The listing builds one solid part. Answer for the finished solid, in the listing's coordinates (mm). A direction names the side the tool comes from. Coordinates: 2 decimals unless noted, no trailing zeros. Loops run counter-clockwise (first coordinate to the right, second up) from the corner with the lowest first, then second, coordinate; pieces in that order, holes last. Notation, with made-up numbers: (32, 44) - (83, 44) arc R20 ccw to (83, 64) - close; hole circle Ø4 at (-8.5, 17.5). An arc over 180 degrees is marked (long way). One line per question, with ' | ' between items.
Autodesk Inventor part; units mm, degrees
ref_plane "YZ Plane" through (0, 0, 0) normal (1, 0, 0) x (0, 1, 0)
ref_plane "XZ Plane" through (0, 0, 0) normal (0, 1, 0) x (-1, 0, 0)
ref_plane "XY Plane" through (0, 0, 0) normal (0, 0, 1) x (1, 0, 0)
sketch "Skizze1" plane through (0, 0, 0) normal (0, 0, 1) x (1, 0, 0)
  line L0 (49.5001, 248.3761) -> (-49.5001, 248.3761)
  line L1 (49.5001, 95.1751) -> (49.5001, 248.3761)
  line L2 (-49.5001, 248.3761) -> (-49.5001, 95.1751) construction
  line L3 (-49.5001, 95.1751) -> (49.5001, 95.1751) construction
  line L4 (49.5001, 95.1751) -> (-20.5915, 95.1751)
  line L5 (-20.5915, 95.1751) -> (-49.5001, 124.0836)
  line L6 (-49.5001, 124.0836) -> (-49.5001, 248.3761)
  line L7 (-39.5001, 238.3761) -> (39.5001, 238.3761)
  line L8 (39.5001, 238.3761) -> (39.5001, 105.1751)
  line L9 (39.5001, 105.1751) -> (-19.2778, 105.1751)
  line L10 (-19.2778, 105.1751) -> (-39.5001, 125.3973)
  line L11 (-39.5001, 125.3973) -> (-39.5001, 238.3761)
  circle A0 centre (44.5001, 243.3761) radius 2.5
  circle A1 centre (-44.5001, 243.3761) radius 2.5
  circle A2 centre (-44.5001, 171.4345) radius 2.5
  circle A3 centre (44.5001, 171.4345) radius 2.5
  circle A4 centre (44.5001, 100.1751) radius 2.5
  circle A5 centre (-20.9666, 110.5265) radius 1.75
  circle A6 centre (-24.6237, 114.0565) radius 1.75
  circle A7 centre (-44.8001, 100.0237) radius 1.75
  circle A8 centre (-29.7001, 100.0237) radius 1.75
  point P0 (0, 0)
  dimension "d0" = 135
  dimension "d1" = 8
  dimension "d3" = 10
  dimension "d4" = 10
  dimension "d5" = 10
  dimension "d6" = 10
  dimension "d22" = 2.5
extrude "Extrusion1" add sketch "Skizze1" along normal blind 1.5 contours L1 L4 L5 L6 L0 | A0 | A1 | A2 | A3 | A4
sketch "Skizze2" plane through (0, 0, 0) normal (0, 0, -1) x (-1, 0, 0)
  circle A0 centre (-44.5001, 100.1751) radius 2.5
  circle A1 centre (-44.5001, 171.4345) radius 2.5
  circle A2 centre (-44.5001, 243.3761) radius 2.5
  circle A3 centre (40.1569, 120.3973) radius 2.5
  circle A4 centre (44.5001, 171.4345) radius 2.5
  circle A5 centre (44.5001, 243.3761) radius 2.5
  circle A6 centre (-44.5001, 100.1751) radius 2.4
  circle A7 centre (-44.5001, 171.4345) radius 2.4
  circle A8 centre (-44.5001, 243.3761) radius 2.4
  circle A9 centre (44.5001, 243.3761) radius 2.4
  circle A10 centre (44.5001, 171.4345) radius 2.4
  circle A11 centre (40.1569, 120.3973) radius 2.4
  dimension "d23" = 0.1
  dimension "d24" = 4.8
  dimension "d25" = 4.8
  dimension "d26" = 4.8
  dimension "d27" = 4.8
  dimension "d28" = 4.8
  dimension "d29" = 4.8
extrude "Extrusion2" add sketch "Skizze2" along normal blind 2.6 contours A6 | A7 | A8 | A9 | A10 | A11
sketch "Skizze3" plane through (0, 0, 0) normal (0, 0, -1) x (-1, 0, 0)
  line L0 (-49.5001, 95.1751) -> (-49.5001, 248.3761)
  line L1 (-39.5001, 238.3761) -> (-39.5001, 105.1751)
  line L2 (-49.5001, 135.1751) -> (-39.5001, 135.1751)
  line L3 (-39.5001, 135.1751) -> (-39.5001, 145.1751)
  line L4 (-39.5001, 145.1751) -> (-49.5001, 145.1751)
  line L5 (-49.5001, 145.1751) -> (-49.5001, 135.1751)
  line L6 (39.5001, 238.3761) -> (39.5001, 125.3973)
  line L7 (49.5001, 248.3761) -> (49.5001, 124.0836)
  line L8 (39.5001, 135.1751) -> (49.5001, 135.1751)
  line L9 (49.5001, 135.1751) -> (49.5001, 145.1751)
  line L10 (49.5001, 145.1751) -> (39.5001, 145.1751)
  line L11 (39.5001, 145.1751) -> (39.5001, 135.1751)
  line L12 (39.5001, 125.3973) -> (19.2778, 105.1751)
  line L13 (20.692, 106.5893) -> (26.3489, 100.9324)
  line L14 (49.5001, 124.0836) -> (20.5915, 95.1751)
  line L15 (26.3489, 100.9324) -> (33.42, 108.0035)
  line L16 (33.42, 108.0035) -> (27.7631, 113.6604)
  line L17 (27.7631, 113.6604) -> (20.692, 106.5893)
  line L18 (20.5915, 95.1751) -> (-49.5001, 95.1751)
  point P0 (0, 0)
  dimension "d11" = 10
  dimension "d12" = 10
  dimension "d13" = 10
  dimension "d14" = 0
  dimension "d15" = 40
  dimension "d16" = 2
extrude "Extrusion3" cut sketch "Skizze3" against normal blind 1 contours L0 L4 L1 L2 | L13 L12 L16 L14 | L8 L6 L10 L7
equation "\"d4\" = d3"
equation "\"d5\" = d3"
equation "\"d6\" = d3"
equation "\"d25\" = d24"
equation "\"d26\" = d24"
equation "\"d27\" = d24"
equation "\"d28\" = d24"
equation "\"d29\" = d24"
equation "\"d12\" = d11"
equation "\"d13\" = d11"
properties part number "Backplate_V2"
Item 1: Each of these flat-tipped pins is pushed along its axis until it touches: pin 1 Ø6.5 at (x, y) = (-34.5, 118.5) entering from -Z; pin 2 Ø3 at (x, y) = (-46.5, 138.5) entering from -Z; pin 3 Ø0.5 at (x, z) = (-46, 0.5) entering from -Y. Where does it stop, or does it pass through?
Taken from the geometry:
pin 1: stops at z = 0 | pin 2: stops at z = 1 | pin 3: stops at y = 120.33
Item 2: Find section C-C, the plane z = -1.4. Write down the section's boundary in (x, y).
Taken from the geometry:
outline: circle Ø4.8 at (-44.5, 171.43); circle Ø4.8 at (-44.5, 243.38); circle Ø4.8 at (-40.16, 120.4); circle Ø4.8 at (44.5, 100.18); circle Ø4.8 at (44.5, 171.43); circle Ø4.8 at (44.5, 243.38)
Item 3: Find the intervals of material crossed by line 1 (X direction, y = 168, z = 0.7); line 2 (Y direction, x = -1, z = 1.05); line 3 (Y direction, x = -44.5, z = 0.45), in increasing order. Write a range as [from, to].
Taken from the geometry:
line 1: x = [-49.5, -39.5], [39.5, 49.5] | line 2: y = [95.18, 105.18], [238.38, 248.38] | line 3: y = [119.08, 135.18], [145.18, 248.38]
Item 4: Find section D-D, the plane x = -23. Write down the section's boundary in (y, z), plus the area to 3 significant figures.
Taken from the geometry:
outline: (97.58, 0) - (104.28, 0) - (104.28, 1) - (108.9, 1) - (108.9, 1.5) - (97.58, 1.5) - close; (238.38, 0) - (248.38, 0) - (248.38, 1.5) - (238.38, 1.5) - close | area: 27.4 mm2
Item 5: The mould has two halves that part along X. Classify faces 5 (the face through (-27, 107, 1)), 6 (the face through (-23.48, 103.8, 0.49)), 7 (the face through (-44, 243, -2.6)): pulls with the +X half, pulls with the -X half, needs draft (parallel to the pull), parting line crosses it, or undercut.
Taken from the geometry:
face 5: undercut | face 6: pulls with the -X half | face 7: needs draft
Item 6: Find section B-B, the plane x = 2.5. Write down the section's boundary in (y, z), plus the area to 3 significant figures.
Taken from the geometry:
outline: (95.18, 0) - (105.18, 0) - (105.18, 1.5) - (95.18, 1.5) - close; (238.38, 0) - (248.38, 0) - (248.38, 1.5) - (238.38, 1.5) - close | area: 30.0 mm2
Item 7: Find section A-A, the plane y = 139.5. Write down the section's boundary in (x, z), plus the area to 3 significant figures.
Taken from the geometry:
outline: (-49.5, 1) - (-39.5, 1) - (-39.5, 1.5) - (-49.5, 1.5) - close; (39.5, 1) - (49.5, 1) - (49.5, 1.5) - (39.5, 1.5) - close | area: 10.0 mm2
Item 8: Which of the six approach directions +Z, -Z, +X, -X, +Y, -Y give full straight-line access (tool end or side, diameter ignored) to faces 1 (the face through (-31.5, 117.4, 0.7)), 2 (the face through (-30.631, 110.792, 0.493)), 3 (the face through (42.211, 99.454, -1.282)), 4 (the face through (45, 243, -2.6))?
Taken from the geometry:
face 1: +Z, -Z | face 2: -Z, -Y | face 3: -Z | face 4: -Z, +X, -X, +Y, -Y
